from build123d import *

# Parameters (mm, degrees)
F0_W          = 160
F0_H          = 120
F1_DEPTH      = 5
F2_R          = 5
F4_DEPTH      = 160
F5_W          = 90
F5_H          = 15
F5_W_2        = 5
F6_DEPTH      = 25
F6_DEPTH_BACK = 25


with BuildPart() as f1:
    # F0 (on Top) → F1 (new body)
    with BuildSketch(Plane.XY):
        Rectangle(F0_W, F0_H)
    extrude(amount=F1_DEPTH)

    # F2
    f2_edges = [f1.edges().sort_by_distance(p)[0] for p in [
        (80, 60, 2.5),
        (80, -60, 2.5),
        (-80, -60, 2.5),
        (-80, 60, 2.5),
    ]]
    fillet(f2_edges, radius=F2_R)

    # F3 (on face) → F4 (join)
    with BuildSketch(Plane.YZ.offset(80)):
        Polygon((9.97, 0), (-9.98, 0), (-14.98, -9.95), (14.97, -9.95), align=None)
    extrude(amount=-F4_DEPTH)

    # F5 (on Front) → F6 (cut, two sides)
    with BuildSketch(Plane.XZ) as f6_sk:
        with Locations((0, -7.5)):
            Rectangle(F5_W, F5_H)
        with Locations((-77.5, -7.5)):
            Rectangle(F5_W_2, F5_H)
        with Locations((77.5, -7.5)):
            Rectangle(F5_W_2, F5_H)
    extrude(amount=F6_DEPTH, mode=Mode.SUBTRACT)
    extrude(f6_sk.sketch, amount=-F6_DEPTH_BACK, mode=Mode.SUBTRACT)


solid = f1.part
The model under review builds one solid part; all positions refer to its coordinate system, in mm. A direction names the side the tool comes from. Round coordinates to 2 decimals unless told otherwise and drop trailing zeros. Order: outer loops, then holes, each group sorted by start corner. A loop starts at its lowest first (then second) coordinate and runs counter-clockwise, first axis right, second up. Notation, with made-up numbers: (-18.75, 37.5) -> (21.25, 37.5) arc R5 ccw to (21.25, 41.5) -> close; hole circle Ø5 at (59, 82). An arc over 180 degrees is marked (long way). Return JSON: item names as keys, results as strings.
1. Take a section at A-A (y = 0). Write out the cut boundary in (x, z).
Answer block:
{"outline": "(-80, 0) -> (-75, 0) -> (-75, -9.95) -> (-45, -9.95) -> (-45, 0) -> (45, 0) -> (45, -9.95) -> (75, -9.95) -> (75, 0) -> (80, 0) -> (80, 5) -> (-80, 5) -> close"}
2. Take a section at B-B (z = -8.25). Write out the cut boundary in (x, y).
Answer block:
{"outline": "(-75, -14.13) -> (-45, -14.13) -> (-45, 14.12) -> (-75, 14.12) -> close; (45, -14.13) -> (75, -14.13) -> (75, 14.12) -> (45, 14.12) -> close"}
3. Take a section at C-C (x = -54). Write out the cut boundary in (y, z), then the cut area to 3 significant figures.
Answer block:
{"outline": "(-60, 0) -> (-9.98, 0) -> (-14.98, -9.95) -> (14.97, -9.95) -> (9.97, 0) -> (60, 0) -> (60, 5) -> (-60, 5) -> close", "area": "848 mm²"}
4. For faces 5 (the face through (45, 0, -5)), 6 (the face through (-75, 0, -5)), 7 (the face through (75, 0, -5)), 8 (the face through (60.21, -12.445, -4.905)), list the 3-axis set-ups (+Z, -Z, +X, -X, +Y, -Y) from which the entire face can be reached by the end or side of a thin tool; tool diameter is ignored.
Answer block:
{"face 5": "-Z, +Y, -Y", "face 6": "-Z, -X, +Y, -Y", "face 7": "-Z, +X, +Y, -Y", "face 8": "+X, -X, -Y"}
5. For L1, parallel to X at y = -4.5, z = -3.5; L2, parallel to Z at x = 19, y = -11; L3, parallel to Y at x = 53, z = -3.5, list the stretches that pass through material, from the lowest coordinate up. Write a range as [from, to].
Answer block:
{"L1": "x = [-75, -45], [45, 75]", "L2": "z = [0, 5]", "L3": "y = [-11.74, 11.73]"}
6. The part is to be moulded in two halves that separate along Z. For faces 1 (the face through (-1, -60, 2)), 2 (the face through (-59.79, -12.445, -4.905)), 3 (the face through (60, 0, -9.95)), 4 (the face through (-59.79, 12.505, -5.045)), say which applies: +Z half, -Z half, draft (parallel to the pull), parting line (faces both ways), or undercut.
Answer block:
{"face 1": "draft", "face 2": "undercut", "face 3": "-Z half", "face 4": "undercut"}
7. Insertion check: P1, Ø5, axis at y = -5.5, z = -4, coming from the +X side; P2, Ø5, axis at y = -2.5, z = -7, coming from the -X side; P3, Ø1.5, axis at y = 40, z = -0.5, coming from the +X side. Each pin has a flat end and moves straight along its axis. Give the tip position at first contact, or say it passes through.
Answer block:
{"P1": "stops at x = 75", "P2": "stops at x = -75", "P3": "stops at x = 80"}
8. Take a section at D-D (y = -28). Write out the cut boundary in (x, z), then the cut area to 3 significant figures.
Answer block:
{"outline": "(-80, 0) -> (80, 0) -> (80, 5) -> (-80, 5) -> close", "area": "800 mm²"}
